Autodesk Inventor part; units mm, degrees
ref_plane "YZ Plane" through (0, 0, 0) normal (1, 0, 0) x (0, 1, 0)
ref_plane "XZ Plane" through (0, 0, 0) normal (0, 1, 0) x (-1, 0, 0)
ref_plane "XY Plane" through (0, 0, 0) normal (0, 0, 1) x (1, 0, 0)
sketch "Skizze1" plane through (0, 0, 0) normal (0, 0, 1) x (1, 0, 0)
  line L0 (0, 7) -> (0, -7) construction
  line L1 (-10.9, 0) -> (30.4, 0) construction
  circle A0 centre (0, 0) radius 2
  circle A1 centre (16, 0) radius 1
  circle A2 centre (19, 0) radius 1
  circle A3 centre (22, 0) radius 1
  arc A4 (22.2841, -2.4838) -> (22.2841, 2.4838) centre (22, 0) ccw
  arc A5 (0.5682, 4.9676) -> (0.5682, -4.9676) centre (0, 0) ccw
  line L2 (0.5682, 4.9676) -> (22.2841, 2.4838)
  line L3 (0.5682, -4.9676) -> (22.2841, -2.4838)
  line L4 (0.5682, -4.9676) -> (0.5682, -1.9176)
  line L5 (0.5682, 1.9176) -> (0.5682, 4.9676)
  line L6 (0.5682, 1.9176) -> (0.5682, -1.9176)
  dimension "d1" = 19
  dimension "d2" = 22
  dimension "d3" = 5
  dimension "d4" = 2
  dimension "d5" = 4
  dimension "d6" = 10
  dimension "d16" = 16
extrude "Extrusion1" add sketch "Skizze1" along normal blind 3
extrude "Extrusion2" add sketch "Skizze1" along normal blind 5 contours L6 A0 | A0 L4 A5 L5 picked at (-0.8876, -0.1748)
chamfer "Fase1" distance 10 distance2 2 1 edges at (0.5682, 0, 3) measured on face at (5.3788, 0, 3)
extrude "Extrusion3" cut sketch "Skizze1" along normal blind 5 contours A0 L6 | L6 A0
properties part number "ServoArm 22mm"
The model under review builds one solid part; all positions refer to its coordinate system, in mm. A direction names the side the tool comes from. Round coordinates to 2 decimals unless told otherwise and drop trailing zeros. Loops run counter-clockwise (first coordinate to the right, second up) from the corner with the lowest first, then second, coordinate; pieces in that order, holes last. Notation, with made-up numbers: M 37,63.25 L 85,63.25 A8 ccw 85,75.25 Z; hole C 66,77 d3. An arc over 180 degrees is marked long. Answer as CSV lines item,"result".
1. We need section A-A (z = 1.5). Give the boundary of the cut face in (x, y), plus the area to 3 significant figures.
Outcome:
outline,"M 0.57,-4.97 L 22.28,-2.48 A2.5 ccw 22.28,2.48 L 0.57,4.97 A5 ccw long Z; hole C 0,0 d4; hole C 16,0 d2; hole C 19,0 d2; hole C 22,0 d2"
area,"193 mm2"
2. We need section B-B (x = 0). Give the boundary of the cut face in (y, z).
Outcome:
outline,"M -5,0 L -2,0 L -2,5 L -5,5 Z; M 2,0 L 5,0 L 5,5 L 2,5 Z"
3. We need section C-C (y = 1.5). Give the boundary of the cut face in (x, z), plus the area to 3 significant figures.
Outcome:
outline,"M -4.77,0 L -1.32,0 L -1.32,5 L -4.77,5 Z; M 1.32,0 L 24,0 L 24,3 L 10.57,3 L 1.32,4.85 Z"
area,"93.8 mm2"
4. Insertion check: pin 1 Ø1 at (x, y) = (16, 3.5) entering from +Z; pin 2 Ø3 at (x, z) = (17, 0.5) entering from +Y; pin 3 Ø3 at (x, z) = (3, 1) entering from +Y; pin 4 Ø4 at (x, y) = (1, 3.5) entering from +Z. Each pin has a flat end and moves straight along its axis. Give the tip position at first contact, or say it passes through.
Outcome:
pin 1,"stops at z = 3"
pin 2,"stops at y = 3.26"
pin 3,"stops at y = 4.86"
pin 4,"stops at z = 5"
5. To check wall thickness, follow L1, parallel to Y at x = 0, z = 0.2; L2, parallel to X at y = -0.5, z = 1.95; L3, parallel to Y at x = -1.5, z = 0.45. State the ranges of each line that lie inside material, in increasing order. Write a range as [from, to].
Outcome:
L1,"y = [-5, -2], [2, 5]"
L2,"x = [-4.97, -1.94], [1.94, 15.13], [16.87, 18.13], [19.87, 21.13], [22.87, 24.45]"
L3,"y = [-4.77, -1.32], [1.32, 4.77]"
6. For faces 5 (the face through (17.4, 0.1, 3)), 6 (the face through (8.86, 4.02, 1.91)), list the 3-axis set-ups (+Z, -Z, +X, -X, +Y, -Y) from which the entire face can be reached by the end or side of a thin tool; tool diameter is ignored.
Outcome:
face 5,"+Z, +X, +Y, -Y"
face 6,"+Z, -Z, +X, +Y"
7. Draft analysis for pull direction Y (two halves, no side actions). For faces 1 (the face through (8.86, -4.02, 1.91)), 2 (the face through (21, 0, 1)), 3 (the face through (17, 0, 1)), 4 (the face through (-5, 0, 2)), state which applies: pulls with the +Y half, pulls with the -Y half, needs draft (parallel to the pull), parting line crosses it, or undercut.
Outcome:
face 1,"pulls with the -Y half"
face 2,"undercut"
face 3,"undercut"
face 4,"parting line crosses it"
